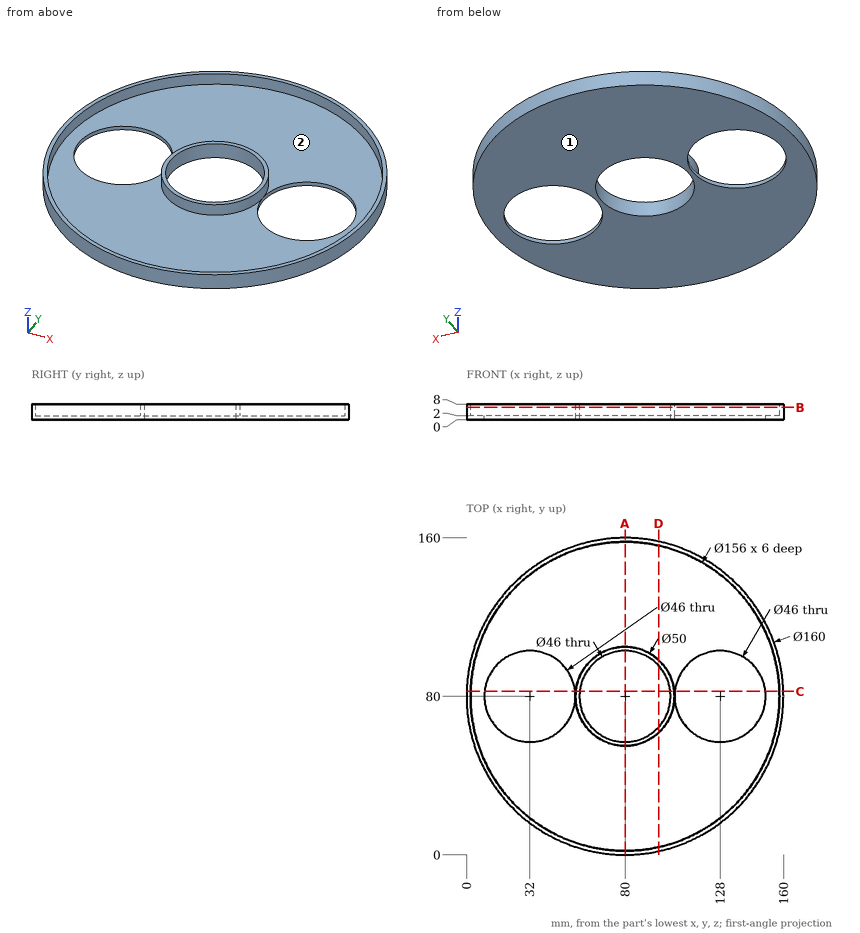
Geometry: see drawing. Coordinates: mm, zero at the bounding-box minimum. Give positions to 0.01 mm unless a question says otherwise; leave off trailing zeros. Loops run counter-clockwise (first coordinate to the right, second up) from the corner with the lowest first, then second, coordinate; pieces in that order, holes last. Notation, with made-up numbers: (69.25, -32) -> (79.25, -32) arc R28 ccw to (79.25, -7) -> close; hole circle Ø8 at (30.5, 79.5). An arc over 180 degrees is marked (long way). Use one line per item in the form item = value.
Item 1: Line query: probe 1 along Y at (x, z) = (80, 4.25); probe 2 along X at (y, z) = (87, 5.25); probe 3 along Y at (x, z) = (76, 2.5). Output: solid intervals per line, ascending.
A:
probe_1 = 0 to 2, 55 to 57, 103 to 105, 158 to 160
probe_2 = 0.31 to 2.31, 56 to 58.09, 101.91 to 104, 157.69 to 159.69
probe_3 = 0.1 to 2.1, 55.32 to 57.35, 102.65 to 104.68, 157.9 to 159.9
Item 2: Section query A-A on x = 80. Output: boundary loops of the cut face in (y, z).
A:
outline = (0, 0) -> (57, 0) -> (57, 8) -> (55, 8) -> (55, 2) -> (2, 2) -> (2, 8) -> (0, 8) -> close; (103, 0) -> (160, 0) -> (160, 8) -> (158, 8) -> (158, 2) -> (105, 2) -> (105, 8) -> (103, 8) -> close
Item 3: Section query D-D on x = 97. Output: boundary loops of the cut face in (y, z), and give its area (3 significant figures).
A:
outline = (1.83, 0) -> (64.51, 0) -> (64.51, 8) -> (61.67, 8) -> (61.67, 2) -> (3.88, 2) -> (3.88, 8) -> (1.83, 8) -> close; (95.49, 0) -> (158.17, 0) -> (158.17, 8) -> (156.12, 8) -> (156.12, 2) -> (98.33, 2) -> (98.33, 8) -> (95.49, 8) -> close
area = 309 mm^2
Item 4: Pin query (flat end, axial travel): P1, Ø4, axis at y = 27, z = 2.5, coming from the -X side; P2, Ø6, axis at x = 71, y = 21.5, coming from the +Z side. Return the tip coordinate at first contact, or that it passes through.
A:
P1 = 18.36
P2 = 2
Item 5: Draft query along X for the marked faces 1 and 2. Return one class per face: pulls with the +X half, pulls with the -X half, needs draft (parallel to the pull), parting line crosses it, or undercut.
A:
face_1 = needs draft
face_2 = undercut
Item 6: Section query B-B on z = 6.25. Output: boundary loops of the cut face in (x, y).
A:
outline = circle Ø160 at (80, 80); circle Ø50 at (80, 80); hole circle Ø156 at (80, 80); hole circle Ø46 at (80, 80)
Item 7: Section query C-C on y = 82.5. Output: boundary loops of the cut face in (x, z), and give its area (3 significant figures).
A:
outline = (0.04, 0) -> (9.14, 0) -> (9.14, 2) -> (2.04, 2) -> (2.04, 8) -> (0.04, 8) -> close; (54.86, 0) -> (57.14, 0) -> (57.14, 8) -> (55.13, 8) -> (55.13, 2) -> (54.86, 2) -> close; (102.86, 0) -> (105.14, 0) -> (105.14, 2) -> (104.87, 2) -> (104.87, 8) -> (102.86, 8) -> close; (150.86, 0) -> (159.96, 0) -> (159.96, 8) -> (157.96, 8) -> (157.96, 2) -> (150.86, 2) -> close
area = 93.6 mm^2
